from build123d import *

# Parameters (mm, degrees)
BOSS_EXTRUDE1_DEPTH = 710
SKETCH2_R           = 3.75
CUT_EXTRUDE1_DEPTH  = 5.3
SKETCH3_R           = 2.25
CUT_EXTRUDE2_DEPTH  = 711.198035762


with BuildPart() as part:
    # Sketch1 → Boss-Extrude1 (new body)
    with BuildSketch(Plane.XY):
        Polygon((-7.5, 0), (7.5, 0), (7.5, 4), (5.5, 6), (5.5, 9), (7.5, 11), (7.5, 15), (-7.5, 15), (-7.5, 11), (-5.5, 9), (-5.5, 6), (-7.5, 4), align=None)
    extrude(amount=BOSS_EXTRUDE1_DEPTH)

    # Sketch2 → Cut-Extrude1 (cut)
    with BuildSketch(Plane(origin=(0, 15, 0), x_dir=(1, 0, 0), z_dir=(0, 1, 0))):
        with Locations(Location((0, -20, 0), (0, 0, 270))):
            Circle(SKETCH2_R)
        with Locations(Location((0, -80, 0), (0, 0, 270))):
            Circle(SKETCH2_R)
        with Locations(Location((0, -140, 0), (0, 0, 270))):
            Circle(SKETCH2_R)
        with Locations(Location((0, -200, 0), (0, 0, 270))):
            Circle(SKETCH2_R)
        with Locations(Location((0, -260, 0), (0, 0, 270))):
            Circle(SKETCH2_R)
    cut_extrude1 = extrude(amount=-CUT_EXTRUDE1_DEPTH, mode=Mode.SUBTRACT)

    # Sketch3 → Cut-Extrude2 (cut, through all)
    with BuildSketch(Plane(origin=(0, 15, 0), x_dir=(1, 0, 0), z_dir=(0, 1, 0))):
        with Locations(Location((0, -20, 0), (0, 0, 270))):
            Circle(SKETCH3_R)
        with Locations(Location((0, -80, 0), (0, 0, 270))):
            Circle(SKETCH3_R)
        with Locations(Location((0, -140, 0), (0, 0, 270))):
            Circle(SKETCH3_R)
        with Locations(Location((0, -200, 0), (0, 0, 270))):
            Circle(SKETCH3_R)
        with Locations(Location((0, -260, 0), (0, 0, 270))):
            Circle(SKETCH3_R)
    extrude(amount=-CUT_EXTRUDE2_DEPTH, mode=Mode.SUBTRACT)

    # 镜向1: Cut-Extrude1 across plane
    add(cut_extrude1.mirror(Plane.XY.offset(355)), mode=Mode.SUBTRACT)


solid = part.part
The listing builds one solid part. Answer for the finished solid, in the listing's coordinates (mm). Coordinates: 2 decimals unless noted, no trailing zeros. Order: outer loops, then holes, each group sorted by start corner. A loop starts at its lowest first (then second) coordinate and runs counter-clockwise, first axis right, second up. Notation, with made-up numbers: (3.5, 58.25) -> (42.5, 58.25) arc R19 ccw to (42.5, 80.25) -> close; hole circle Ø11 at (4, 84). An arc over 180 degrees is marked (long way). Answer in a Markdown table with one row per item. Add a question column.
Item 1: Each of these flat-tipped pins is pushed along its axis until it touches: P1, Ø3, axis at y = 9, z = 229.5, coming from the +X side; P2, Ø5, axis at x = 0, z = 80, coming from the +Y side; P3, Ø2.5, axis at y = 7, z = 250.5, coming from the +X side. Where does it stop, or does it pass through?
Item 2: Find the intervals of material crossed by L1, parallel to X at y = 13.4, z = 140; L2, parallel to Z at x = 1.5, y = 8; L3, parallel to Z at x = 0.75, y = 8.5, in increasing order. Write a range as from..to.
Item 3: Find section A-A (z = 184.5). Write down the section's boundary in (x, y), then the cut area to 3 significant figures.
Result set:
| question | item | result |
|---|---|---|
| 1 | P1 | stops at x = 7 |
| 1 | P2 | stops at y = 9.7 |
| 1 | P3 | stops at x = 5.75 |
| 2 | L1 | x = -7.5..-3.75, 3.75..7.5 |
| 2 | L2 | z = 0..18.32, 21.68..78.32, 81.68..138.32, 141.68..198.32, 201.68..258.32, 261.68..710 |
| 2 | L3 | z = 0..17.88, 22.12..77.88, 82.12..137.88, 142.12..197.88, 202.12..257.88, 262.12..710 |
| 3 | outline | (-7.5, 0) -> (7.5, 0) -> (7.5, 4) -> (5.5, 6) -> (5.5, 9) -> (7.5, 11) -> (7.5, 15) -> (-7.5, 15) -> (-7.5, 11) -> (-5.5, 9) -> (-5.5, 6) -> (-7.5, 4) -> close |
| 3 | area | 205 mm² |
